Autodesk Inventor part; units mm, degrees
ref_plane "left_XY" through (0, 0, 0) normal (0, 0, 1) x (1, 0, 0)
ref_plane "left_YZ" through (0, 0, 0) normal (1, 0, 0) x (0, 1, 0)
ref_plane "left_ZX" through (0, 0, 0) normal (0, 1, 0) x (0, 0, 1)
sketch "Sketch_1" plane through (0, 0, 0) normal (0, 0, 1) x (1, 0, 0)
  line L0 (-10.597, 2.9503) -> (-8.764, 1.4122)
  arc A0 (-8.764, -1.4122) -> (-8.764, 1.4122) centre (-10.005, 0) ccw
  line L1 (-8.764, -1.4122) -> (-10.4531, -3.4252)
  arc A1 (-10.4531, -3.4252) -> (-9.5793, -5.4071) centre (0, 0) ccw
  line L2 (-9.5793, -5.4071) -> (-7.1956, -5.1985)
  arc A2 (-5.1985, -7.1956) -> (-7.1956, -5.1985) centre (-7.0746, -7.0746) ccw
  line L3 (-5.1985, -7.1956) -> (-4.9695, -9.8135)
  arc A3 (-4.9695, -9.8135) -> (-2.9503, -10.597) centre (0, 0) ccw
  line L4 (-2.9503, -10.597) -> (-1.4122, -8.764)
  arc A4 (1.4122, -8.764) -> (-1.4122, -8.764) centre (0, -10.005) ccw
  line L5 (1.4122, -8.764) -> (3.4252, -10.4531)
  arc A5 (3.4252, -10.4531) -> (5.4071, -9.5793) centre (0, 0) ccw
  line L6 (5.4071, -9.5793) -> (5.1985, -7.1956)
  arc A6 (7.1956, -5.1985) -> (5.1985, -7.1956) centre (7.0746, -7.0746) ccw
  line L7 (7.1956, -5.1985) -> (9.8135, -4.9695)
  arc A7 (9.8135, -4.9695) -> (10.597, -2.9503) centre (0, 0) ccw
  line L8 (10.597, -2.9503) -> (8.764, -1.4122)
  arc A8 (8.764, 1.4122) -> (8.764, -1.4122) centre (10.005, 0) ccw
  line L9 (8.764, 1.4122) -> (10.4531, 3.4252)
  arc A9 (10.4531, 3.4252) -> (9.5793, 5.4071) centre (0, 0) ccw
  line L10 (9.5793, 5.4071) -> (7.1956, 5.1985)
  arc A10 (5.1985, 7.1956) -> (7.1956, 5.1985) centre (7.0746, 7.0746) ccw
  line L11 (5.1985, 7.1956) -> (4.9695, 9.8135)
  arc A11 (4.9695, 9.8135) -> (2.9503, 10.597) centre (0, 0) ccw
  line L12 (2.9503, 10.597) -> (1.4122, 8.764)
  arc A12 (-1.4122, 8.764) -> (1.4122, 8.764) centre (0, 10.005) ccw
  line L13 (-1.4122, 8.764) -> (-3.4252, 10.4531)
  arc A13 (-3.4252, 10.4531) -> (-5.4071, 9.5793) centre (0, 0) ccw
  line L14 (-5.4071, 9.5793) -> (-5.1985, 7.1956)
  arc A14 (-7.1956, 5.1985) -> (-5.1985, 7.1956) centre (-7.0746, 7.0746) ccw
  line L15 (-7.1956, 5.1985) -> (-9.8135, 4.9695)
  arc A15 (-9.8135, 4.9695) -> (-10.597, 2.9503) centre (0, 0) ccw
extrude "Extrusion1" add sketch "Sketch_1" along normal blind 17
sketch "Sketch2" plane through (0, 0, 0) normal (0, 0, -1) x (-1, 0, 0)
  point P0 (0, 0)
hole "Hole1" at (0, 0, 0) direction (0, 0, 1) diameter 10 depth 17
ref_plane "left_XY" through (0, 0, 0) normal (0, 0, 1) x (1, 0, 0)
ref_plane "left_YZ" through (0, 0, 0) normal (1, 0, 0) x (0, 1, 0)
ref_plane "left_ZX" through (0, 0, 0) normal (0, 1, 0) x (0, 0, 1)
ref_plane "right_XY" through (0, 0, 17) normal (0, 0, 1) x (1, 0, 0)
ref_plane "right_YZ" through (0, 0, 17) normal (1, 0, 0) x (0, 1, 0)
ref_plane "right_ZX" through (0, 0, 17) normal (0, 1, 0) x (0, 0, 1)
properties part number "MSF-25 Sleeve"
Build history of the part. All positions in model axes, mm. A direction names the side the tool comes from. Round coordinates to 2 decimals unless told otherwise and drop trailing zeros. Write each loop counter-clockwise with the first axis right and the second up, starting at its lowest first coordinate (ties: lowest second). Pieces come first, ordered by that corner, then holes. Notation, with made-up numbers: (19, -4.5) - (30, -4.5) arc R22 ccw to (30, 21.5) - close; hole circle Ø3 at (-10, 2.5). An arc over 180 degrees is marked (long way). Write each question's results on one line, items separated by ' | '. Start each with the question number.
Item 1: Mould opens along X. For faces 1 (the face through (4.88, -1.08, 8.62)), 2 (the face through (-4.45, 10.06, 8.38)), 3 (the face through (5.304, -8.404, 8.381)) say: pulls with the +X half, pulls with the -X half, needs draft (parallel to the pull), parting line crosses it, or undercut.
Item 2: Drop flat-ended pins along their axis: P1, Ø1.5, axis at y = -1.5, z = 2.5, coming from the +X side; P2, Ø3, axis at y = 3, z = 10, coming from the +X side; P3, Ø8, axis at x = -2, z = 13, coming from the -Y side. Give the stop position or say it passes through.
Item 3: Saw through at D-D (x = 7.75). Write the cut outline in (y, z), and give its area (3 significant figures).
Item 4: Wall check: L1, parallel to X at y = 0, z = 5.5 (3 decimals); L2, parallel to Y at x = -1, z = 8.25. Give the ranges that are in metal, low to high. Write a range as [from, to].
Item 5: Which spindle directions (+Z, -Z, +X, -X, +Y, -Y) get a long thin tool onto all of the face, cutting with end or side? Do faces 4 (the face through (9.597, 2.405, 8.381)), 5 (the face through (2.2, 9.7, 8.4)), 6 (the face through (-9.7, 2.2, 8.4)), 7 (the face through (-2.2, -9.7, 8.4)), 8 (the face through (3.97, 10.26, 8.38)). Say none if no direction does.
Item 6: Saw through at A-A (y = 0). Write the cut outline in (x, z) (3 decimals).
Results are:
1) face 1: undercut | face 2: pulls with the -X half | face 3: pulls with the +X half
2) P1: stops at x = 9.76 | P2: stops at x = 10.45 | P3: stops at y = -10.6
3) outline: (-5.15, 0) - (5.25, 0) - (5.25, 17) - (-5.15, 17) - close | area: 177 mm²
4) L1: x = [-8.125, -5], [5, 8.125] | L2: y = [-8.41, -4.9], [4.9, 8.41]
5) face 4: +Z, -Z, +X | face 5: +Z, -Z, +Y | face 6: +Z, -Z, -X | face 7: +Z, -Z, -Y | face 8: +Z, -Z, +X, +Y
6) outline: (-8.125, 0) - (-5, 0) - (-5, 17) - (-8.125, 17) - close; (5, 0) - (8.125, 0) - (8.125, 17) - (5, 17) - close
